The listing builds one solid part. Answer for the finished solid, in the listing's coordinates (mm). A direction names the side the tool comes from. Coordinates: 2 decimals unless noted, no trailing zeros. Loops run counter-clockwise (first coordinate to the right, second up) from the corner with the lowest first, then second, coordinate; pieces in that order, holes last. Notation, with made-up numbers: M 9,71.5 L 41,71.5 A26 ccw 41,102.5 Z; hole C 23,-13.75 d6. An arc over 180 degrees is marked long. Return JSON: item names as keys, results as strings. Group by question number.
1. Section C-C (x = 0) is taken. Write down the section's boundary in (y, z) (3 decimals), then the cut area to 3 significant figures.
2. Straight lines are drawn through the part: L1, parallel to X at y = -0.5, z = 0.25; L2, parallel to Z at x = -5, y = -1; L3, parallel to X at y = 1, z = -2.5. For each, find the intervals that lie inside material, in ascending order. Write a range as from..to.
3. Which of the six approach directions +Z, -Z, +X, -X, +Y, -Y give full straight-line access (tool end or side, diameter ignored) to faces 1 (the face through (-5.5, 0.7, -6.05)), 2 (the face through (3.7, 1, 0)), 3 (the face through (5.5, 0.7, -6.05))?
4. Section B-B (z = 0) is taken. Write down the section's boundary in (x, y) (3 decimals), then the cut area to 3 significant figures.
5. Section A-A (y = 1.25) is taken. Write down the section's boundary in (x, z) (3 decimals).
6. Given P1, Ø0.9, axis at y = -0.5, z = 5.5, coming from the +X side; P2, Ø0.9, axis at x = 6, y = 1.5, coming from the -Z side; P3, Ø7, axis at x = 0, z = 0, coming from the -Y side; P4, Ø6, axis at x = -0.5, z = 1, coming from the +Y side, each flat-ended and moving along its own axis, determine where each tip first touches the part or whether it passes through.
7. Section D-D (y = -0.5) is taken. Write down the section's boundary in (x, z), then the cut area to 3 significant figures.
```python
from build123d import *

# Parameters (mm, degrees)
SKETCH1_W           = 7.4
SKETCH1_H           = 7.4
SKETCH1_R           = 1.375
BOSS_EXTRUDE1_DEPTH = 2
SKETCH2_W           = 12.1
SKETCH2_H           = 12.1
SKETCH2_W_2         = 10.1
SKETCH2_H_2         = 10.1
BOSS_EXTRUDE2_DEPTH = 2
SKETCH3_W           = 12.1
SKETCH3_H           = 12.1
SKETCH3_R           = 2.75
BOSS_EXTRUDE3_DEPTH = 2
SKETCH4_R           = 2.75
SKETCH4_R_2         = 1.675
SKETCH4_R_3         = 1.375
BOSS_EXTRUDE4_DEPTH = 2
SKETCH5_R           = 1.675
BOSS_EXTRUDE5_DEPTH = 1.3
SKETCH10_W          = 12.1
SKETCH10_H          = 12.1
SKETCH10_W_2        = 10.1
SKETCH10_H_2        = 10.1
BOSS_EXTRUDE6_DEPTH = 3.175
SKETCH11_W          = 8.881017399
SKETCH11_H          = 18.09347602
CUT_EXTRUDE1_DEPTH  = 10
BOSS_EXTRUDE7_DEPTH = 6.475


with BuildPart() as part:
    # Sketch1 → Boss-Extrude1 (new body)
    with BuildSketch(Plane(origin=(0, 0, 0), x_dir=(1, 0, 0), z_dir=(0, 1, 0))):
        Rectangle(SKETCH1_W, SKETCH1_H)
        with Locations(Location((0, 0, 0), (0, 0, 270))):
            Circle(SKETCH1_R, mode=Mode.SUBTRACT)
    extrude(amount=BOSS_EXTRUDE1_DEPTH)



with BuildPart() as body_2:
    # Sketch2 → Boss-Extrude2 (new body)
    with BuildSketch(Plane(origin=(0, 2, 0), x_dir=(1, 0, 0), z_dir=(0, 1, 0))):
        Rectangle(SKETCH2_W, SKETCH2_H)
        Rectangle(SKETCH2_W_2, SKETCH2_H_2, mode=Mode.SUBTRACT)
    extrude(amount=-BOSS_EXTRUDE2_DEPTH)


with BuildPart() as part_1:
    add(part.part)

    add(body_2.part)  # Boss-Extrude3 merges body 2
    # Sketch3 → Boss-Extrude3 (add)
    with BuildSketch(Plane(origin=(0, 2, 0), x_dir=(1, 0, 0), z_dir=(0, 1, 0))):
        Rectangle(SKETCH3_W, SKETCH3_H)
        with Locations(Location((0, 0, 0), (0, 0, 270))):
            Circle(SKETCH3_R, mode=Mode.SUBTRACT)
    extrude(amount=BOSS_EXTRUDE3_DEPTH)

    # Sketch4 → Boss-Extrude4 (add)
    # profile 1 of 2: a face of its own
    with BuildSketch(Plane(origin=(0, 2, 0), x_dir=(1, 0, 0), z_dir=(0, 1, 0))):
        with BuildLine():
            Line((4, 0), (4, -20))
            ThreePointArc((4, -20), (0, -24), (-4, -20))
            Line((-4, -20), (-4, 0))
            ThreePointArc((-4, 0), (0, 4), (4, 0))
        make_face()
        with Locations(Location((0, 0, 0), (0, 0, 270))):
            Circle(SKETCH4_R, mode=Mode.SUBTRACT)
        with Locations(Location((0, -20, 0), (0, 0, 270))):
            Circle(SKETCH4_R_2, mode=Mode.SUBTRACT)
    # profile 2 of 2: a face of its own
    with BuildSketch(Plane(origin=(0, 2, 0), x_dir=(1, 0, 0), z_dir=(0, 1, 0))):
        with Locations(Location((0, 0, 0), (0, 0, 270))):
            Circle(SKETCH4_R_3)
    extrude(amount=BOSS_EXTRUDE4_DEPTH)


with BuildPart() as boss_extrude4_kept_piece:
    # of the separate pieces the step leaves, the one the design keeps (boss_extrude4_pieces_kept)
    add(part_1.part.solids().sort_by_distance((-3.7, 0, 3.7))[0])

    # Sketch5 → Boss-Extrude5 (add)
    # profile 1 of 2: a face of its own
    with BuildSketch(Plane(origin=(0, 2, 0), x_dir=(-1, 0, 0), z_dir=(0, -1, 0))):
        with BuildLine():
            ThreePointArc((-4, -20), (0, -16), (4, -20))
            Line((4, -20), (4, -6.05))
            Line((4, -6.05), (-4, -6.05))
            Line((-4, -6.05), (-4, -20))
        make_face()
    # profile 2 of 2: a face of its own
    with BuildSketch(Plane(origin=(0, 2, 0), x_dir=(-1, 0, 0), z_dir=(0, -1, 0))):
        with BuildLine():
            ThreePointArc((-4, -20), (0, -24), (4, -20))
            ThreePointArc((4, -20), (0, -16), (-4, -20))
        make_face()
        with Locations(Location((0, -20, 0), (0, 0, 90))):
            Circle(SKETCH5_R, mode=Mode.SUBTRACT)
    extrude(amount=BOSS_EXTRUDE5_DEPTH)

    # Sketch10 → Boss-Extrude6 (add)
    with BuildSketch(Plane.XZ.offset(-0.7)):
        Rectangle(SKETCH10_W, SKETCH10_H)
        Rectangle(SKETCH10_W_2, SKETCH10_H_2, mode=Mode.SUBTRACT)
    extrude(amount=BOSS_EXTRUDE6_DEPTH)

    # Sketch11 → Cut-Extrude1 (cut)
    with BuildSketch(Plane(origin=(0, 0.7, 0), x_dir=(-1, 0, 0), z_dir=(0, -1, 0))):
        with Locations((-0.4405087, -15.09673801)):
            Rectangle(SKETCH11_W, SKETCH11_H)
    extrude(amount=-CUT_EXTRUDE1_DEPTH, mode=Mode.SUBTRACT)

    # Sketch14 → Boss-Extrude7 (add)
    with BuildSketch(Plane(origin=(0, -2.475, 0), x_dir=(-1, 0, 0), z_dir=(0, -1, 0))):
        with BuildLine():
            Line((-4.923159555, 6.05), (4.923159555, 6.05))
            ThreePointArc((4.923159555, 6.05), (0, 7.8), (-4.923159555, 6.05))
        make_face()
        with BuildLine():
            ThreePointArc((6.05, -4.923159555), (7.8, 0), (6.05, 4.923159555))
            Line((6.05, 4.923159555), (6.05, -4.923159555))
        make_face()
        with BuildLine():
            Line((-6.05, -4.923159555), (-6.05, 4.923159555))
            ThreePointArc((-6.05, 4.923159555), (-7.8, 0), (-6.05, -4.923159555))
        make_face()
        with BuildLine():
            ThreePointArc((-4.923159555, -6.05), (0, -7.8), (4.923159555, -6.05))
            Line((4.923159555, -6.05), (-4.923159555, -6.05))
        make_face()
    extrude(amount=-BOSS_EXTRUDE7_DEPTH)


solid = boss_extrude4_kept_piece.part
```
Worked out:
{
 "1": {"outline": "M -2.475,-7.8 L 4,-7.8 L 4,-2.75 L 2,-2.75 L 2,-1.375 L 0,-1.375 L 0,-3.7 L 2,-3.7 L 2,-5.05 L -2.475,-5.05 Z; M -2.475,5.05 L 2,5.05 L 2,3.7 L 0,3.7 L 0,1.375 L 2,1.375 L 2,2.75 L 4,2.75 L 4,7.8 L -2.475,7.8 Z", "area": "54.1 mm^2"},
 "2": {"L1": "-7.8..-5.05, 5.05..7.8", "L2": "-6.05..-5.05, 5.05..6.05", "L3": "-7.39..-5.05, -3.7..3.7, 5.05..7.39"},
 "3": {"face 1": "-Z, -X, +Y, -Y", "face 2": "-Y", "face 3": "-Z, +X, +Y, -Y"},
 "4": {"outline": "M -7.8,-2.475 L -5.05,-2.475 L -5.05,2 L -3.7,2 L -3.7,0 L -1.375,0 L -1.375,2 L -2.75,2 L -2.75,4 L -7.8,4 Z; M 1.375,0 L 3.7,0 L 3.7,2 L 5.05,2 L 5.05,-2.475 L 7.8,-2.475 L 7.8,4 L 2.75,4 L 2.75,2 L 1.375,2 Z", "area": "54.1 mm^2"},
 "5": {"outline": "M -6.05,-6.05 L -4.923,-6.05 A7.8 ccw 4.923,-6.05 L 6.05,-6.05 L 6.05,-4.923 A7.8 ccw 6.05,4.923 L 6.05,6.05 L 4.923,6.05 A7.8 ccw -4.923,6.05 L -6.05,6.05 L -6.05,4.923 A7.8 ccw -6.05,-4.923 Z; M -3.7,-3.7 L 3.7,-3.7 L 3.7,3.7 L -3.7,3.7 Z; hole M -5.05,-5.05 L 5.05,-5.05 L 5.05,5.05 L -5.05,5.05 Z; hole C 0,0 d2.75"},
 "6": {"P1": "x = 6.05", "P2": "z = -6.05", "P3": "y = 0", "P4": "y = 4"},
 "7": {"outline": "M -6.05,-6.05 L -4.92,-6.05 A7.8 ccw 4.92,-6.05 L 6.05,-6.05 L 6.05,-4.92 A7.8 ccw 6.05,4.92 L 6.05,6.05 L 4.92,6.05 A7.8 ccw -4.92,6.05 L -6.05,6.05 L -6.05,4.92 A7.8 ccw -6.05,-4.92 Z; hole M -5.05,-5.05 L 5.05,-5.05 L 5.05,5.05 L -5.05,5.05 Z", "area": "91.5 mm^2"}
}
